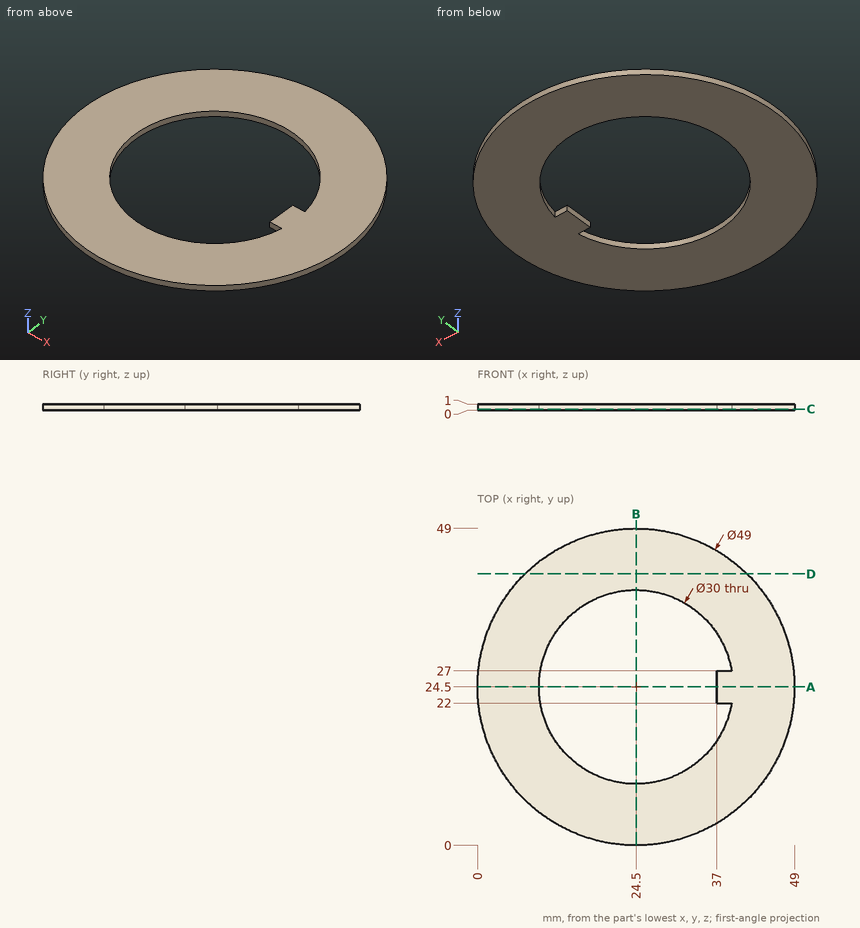
For this review, use the dimensioned drawing (mm, ordinates from the lowest corner) and the shaded views. Round coordinates to 2 decimals unless told otherwise and drop trailing zeros. Order: outer loops, then holes, each group sorted by start corner. A loop starts at its lowest first (then second) coordinate and runs counter-clockwise, first axis right, second up. Notation, with made-up numbers: M -23,7.5 L -15,7.5 A18 ccw -15,37.5 Z; hole C 31.5,75 d11. An arc over 180 degrees is marked long. Use a Markdown table: item, result. Add a question column.
Item 1: To check wall thickness, follow line 1 along X through (y, z) = (24.5, 0.2); line 2 along Y through (x, z) = (24.5, 0.6); line 3 along Y through (x, z) = (36, 0.5). State the ranges of each line that lie inside material, in increasing order.
Item 2: Add section A-A, the plane y = 24.5. Give the boundary of the cut face in (x, z), then the cut area to 3 significant figures.
Item 3: Add section C-C, the plane z = 0.2. Give the boundary of the cut face in (x, y).
Item 4: Add section D-D, the plane y = 42. Give the boundary of the cut face in (x, z).
Item 5: Add section B-B, the plane x = 24.5. Give the boundary of the cut face in (y, z).
Item 6: Insertion check: pin 1 (6 mm diameter, centred on x = 24, y = 11.5, fed in from +Z); pin 2 (0.5 mm diameter, centred on x = 38.5, z = 0.5, fed in from -Y); pin 3 (0.5 mm diameter, centred on y = 25, z = 0.5, fed in from -X). Each pin has a flat end and moves straight along its axis. Give the tip position at first contact, or say it passes through.
Geometry results:
| question | item | result |
|---|---|---|
| 1 | line 1 | x = 0 to 9.5, 37 to 49 |
| 1 | line 2 | y = 0 to 9.5, 39.5 to 49 |
| 1 | line 3 | y = 2.87 to 14.87, 34.13 to 46.13 |
| 2 | outline | M 0,0 L 9.5,0 L 9.5,1 L 0,1 Z; M 37,0 L 49,0 L 49,1 L 37,1 Z |
| 2 | area | 21.5 mm² |
| 3 | outline | C 24.5,24.5 d49; hole M 37,22 L 37,27 L 39.29,27 A15 ccw long 39.29,22 Z |
| 4 | outline | M 7.35,0 L 41.65,0 L 41.65,1 L 7.35,1 Z |
| 5 | outline | M 0,0 L 9.5,0 L 9.5,1 L 0,1 Z; M 39.5,0 L 49,0 L 49,1 L 39.5,1 Z |
| 6 | pin 1 | stops at z = 1 |
| 6 | pin 2 | stops at y = 4.22 |
| 6 | pin 3 | stops at x = 0 |
